Work out the finished part from the listing and answer in its coordinate system (mm). A direction names the side the tool comes from. Round coordinates to 2 decimals unless told otherwise and drop trailing zeros. Write each loop counter-clockwise with the first axis right and the second up, starting at its lowest first coordinate (ties: lowest second). Pieces come first, ordered by that corner, then holes. Notation, with made-up numbers: (64.5, 71.25) - (73.5, 71.25) arc R9 cw to (73.5, 82.25) - close; hole circle Ø6 at (-6, 16). An arc over 180 degrees is marked (long way). Answer as a JSON object with one key per item and string values.
```python
from build123d import *

# Parameters (mm, degrees)
SKETCH003_W    = 0.5
SKETCH003_H    = 0.5
SKETCH003_W_2  = 1
SKETCH003_H_2  = 0.4
PAD002_DEPTH   = 1
SKETCH001_W    = 28
SKETCH001_H    = 5
PAD001_DEPTH   = 15
SKETCH002_W    = 1
SKETCH002_H    = 2
POCKET_DEPTH   = 2
CHAMFER_SIZE   = 1.99
FILLET_R       = 1
FILLET001_R    = 0.25
SKETCH_W       = 0.5
SKETCH_H       = 0.5
SKETCH_W_2     = 1
SKETCH_H_2     = 0.4
PAD_DEPTH      = 1.3
PAD_DEPTH_BACK = 3.5
FILLET003_R    = 0.2


with BuildPart() as pad002:
    # Sketch003 → Pad002 (new body)
    with BuildSketch(Plane(origin=(-3.75, 1, 1.6), x_dir=(1, 0, 0), z_dir=(0, -1, 0))):
        with Locations((0, -0.05)):
            Rectangle(SKETCH003_W, SKETCH003_H)
        with Locations((3.75, -0.05)):
            Rectangle(SKETCH003_W, SKETCH003_H)
        with Locations((15, 0)):
            Rectangle(SKETCH003_W_2, SKETCH003_H_2)
        with Locations((20, 0)):
            Rectangle(SKETCH003_W_2, SKETCH003_H_2)
        with Locations((25, 0)):
            Rectangle(SKETCH003_W_2, SKETCH003_H_2)
    extrude(amount=PAD002_DEPTH)


with BuildPart() as fillet001:
    # Sketch001 → Pad001 (new body)
    with BuildSketch(Plane(origin=(-3.75, 0.6, 1.3), x_dir=(1, 0, 0), z_dir=(0, 1, 0))):
        with Locations((12.9, -1.2)):
            Rectangle(SKETCH001_W, SKETCH001_H)
    extrude(amount=PAD001_DEPTH)

    # Sketch002 → Pocket (cut)
    with BuildSketch(Plane(origin=(-3.75, 15.6, 1.3), x_dir=(1, 0, 0), z_dir=(0, 1, 0))):
        with Locations((18.6, -2.7)):
            Rectangle(SKETCH002_W, SKETCH002_H)
        with Locations((20.6, -2.7)):
            Rectangle(SKETCH002_W, SKETCH002_H)
    extrude(amount=-POCKET_DEPTH, mode=Mode.SUBTRACT)

    # Chamfer
    chamfer_edges = [fillet001.edges().sort_by_distance(p)[0] for p in [
        (16.85, 13.6, 3),
        (14.85, 13.6, 3),
    ]]
    chamfer(chamfer_edges, length=CHAMFER_SIZE)

    # Fillet
    fillet_edges = [fillet001.edges().sort_by_distance(p)[0] for p in [
        (-4.85, 15.6, 2.5),
        (23.15, 15.6, 2.5),
    ]]
    fillet(fillet_edges, radius=FILLET_R)

    # Fillet001
    fillet001_edges = [fillet001.edges().sort_by_distance(p)[0] for p in [
        (-4.85, 7.6, 0),
        (-4.557107, 15.307107, 0),
        (9.15, 0.6, 0),
        (9.15, 15.6, 0),
        (23.15, 7.6, 0),
        (22.857107, 15.307107, 0),
    ]]
    fillet(fillet001_edges, radius=FILLET001_R)


with BuildPart() as obj1:
    # Sketch → Pad (new body, two sides)
    with BuildSketch(Plane(origin=(-3.75, 0, 0.5), x_dir=(1, 0, 0), z_dir=(0, 0, 1))) as pad_sk:
        Rectangle(SKETCH_W, SKETCH_H)
        with Locations((3.75, 0)):
            Rectangle(SKETCH_W, SKETCH_H)
        with Locations((15, 0)):
            Rectangle(SKETCH_W_2, SKETCH_H_2)
        with Locations((20, 0)):
            Rectangle(SKETCH_W_2, SKETCH_H_2)
        with Locations((25, 0)):
            Rectangle(SKETCH_W_2, SKETCH_H_2)
    extrude(amount=PAD_DEPTH)
    extrude(pad_sk.sketch, amount=-PAD_DEPTH_BACK)

    # Fillet003
    fillet003_edges = [obj1.edges().sort_by_distance(p)[0] for p in [
        (-3.75, -0.25, 1.8),
        (0, -0.25, 1.8),
        (11.25, -0.2, 1.8),
        (16.25, -0.2, 1.8),
        (21.25, -0.2, 1.8),
    ]]
    fillet(fillet003_edges, radius=FILLET003_R)

    add(pad002.part)
    add(fillet001.part)


solid = obj1.part
```
Item 1: A cutting plane is placed at D-D (z = 4.25). Write down the section's boundary in (x, y), and give its area (3 significant figures).
Results found:
{"outline": "(-4.85, 0.6) - (23.15, 0.6) - (23.15, 14.6) arc R1 ccw to (22.15, 15.6) - (17.35, 15.6) - (17.35, 14.34) - (16.35, 14.34) - (16.35, 15.6) - (15.35, 15.6) - (15.35, 14.34) - (14.35, 14.34) - (14.35, 15.6) - (-3.85, 15.6) arc R1 ccw to (-4.85, 14.6) - close", "area": "417 mm²"}
Item 2: Determine the mould class of faces 6 (the cylindrical face through (-4.549, 15.315, 2.592)), 7 (the flat face through (11, -0.2, -1)), 8 (the flat face through (16.84, 14.61, 3.98)) for opening direction X: pulls with the +X half, pulls with the -X half, needs draft (parallel to the pull), parting line crosses it, or undercut.
Results found:
{"face 6": "pulls with the -X half", "face 7": "needs draft", "face 8": "undercut"}
Item 3: A cutting plane is placed at B-B (y = 14). Write down the section's boundary in (x, z).
Results found:
{"outline": "(-4.85, 0.25) arc R0.25 ccw to (-4.6, 0) - (22.9, 0) arc R0.25 ccw to (23.15, 0.25) - (23.15, 5) - (17.35, 5) - (17.35, 4.59) - (16.35, 4.59) - (16.35, 5) - (15.35, 5) - (15.35, 4.59) - (14.35, 4.59) - (14.35, 5) - (-4.85, 5) - close"}
Item 4: Each of these flat-tipped pins is pushed along its axis until it touches: P1, Ø4, axis at x = 7.5, z = 3, coming from the -Y side; P2, Ø0.9, axis at y = 0, z = -1, coming from the -X side; P3, Ø3, axis at x = 19, y = 3.5, coming from the -Z side. Where does it stop, or does it pass through?
Results found:
{"P1": "y = 0.6", "P2": "x = -4", "P3": "z = 0"}
Item 5: For faces 1 (the flat face through (21, -0.2, -1)), 2 (the flat face through (-0.25, 0, -1)), 3 (the flat face through (14.84, 14.61, 3.98)), 4 (the flat face through (16, 0.2, -1)), 5 (the flat face through (9, 8, 0)), determine the directions among +Z, -Z, +X, -X, +Y, -Y from which every point of the face is accessible in a straight line to the end or side of a thin tool.
Results found:
{"face 1": "+Z, -Z, +X, -Y", "face 2": "+Z, -Z, -Y", "face 3": "+Z, +Y", "face 4": "-Z, +X", "face 5": "-Z, +X, -X, +Y"}
Item 6: A cutting plane is placed at A-A (z = -0.5). Write down the section's boundary in (x, y), and give its area (3 significant figures).
Results found:
{"outline": "(-4, -0.25) - (-3.5, -0.25) - (-3.5, 0.25) - (-4, 0.25) - close; (-0.25, -0.25) - (0.25, -0.25) - (0.25, 0.25) - (-0.25, 0.25) - close; (10.75, -0.2) - (11.75, -0.2) - (11.75, 0.2) - (10.75, 0.2) - close; (15.75, -0.2) - (16.75, -0.2) - (16.75, 0.2) - (15.75, 0.2) - close; (20.75, -0.2) - (21.75, -0.2) - (21.75, 0.2) - (20.75, 0.2) - close", "area": "1.70 mm²"}
Item 7: Consider line 1 along X through (y, z) = (15, 4); line 2 along Y through (x, z) = (4, 4.5); line 3 along Z through (x, y) = (16.25, 7). Determine where each line is inside the solid, lowest interval first.
Results found:
{"line 1": "-4.77 to 14.35, 15.35 to 16.35, 17.35 to 23.07", "line 2": "0.6 to 15.6", "line 3": "0 to 5"}
Item 8: A cutting plane is placed at C-C (x = 3). Write down the section's boundary in (y, z).
Results found:
{"outline": "(0.6, 0.25) arc R0.25 ccw to (0.85, 0) - (15.35, 0) arc R0.25 ccw to (15.6, 0.25) - (15.6, 5) - (0.6, 5) - close"}
